Input: part model. Units: mm. Frame: model coordinates. Face numbers are marked on the shaded views. A direction names the side the tool comes from. Round coordinates to 2 decimals unless told otherwise and drop trailing zeros. Loops run counter-clockwise (first coordinate to the right, second up) from the corner with the lowest first, then second, coordinate; pieces in that order, holes last. Notation, with made-up numbers: (35.25, -36.75) -> (91.25, -36.75) arc R27 ccw to (91.25, -10.75) -> close; hole circle Ø10 at (-6, 20). An arc over 180 degrees is marked (long way). Answer in a Markdown table with one row per item. Add a question column.
Q1. Pin query (flat end, axial travel): pin 1 (1.4 mm diameter, centred on x = 8.5, y = 13, fed in from +Z). Return the tip coordinate at first contact, or that it passes through.
Q2. Section C-C, the plane x = 24. Output: boundary loops of the cut face in (y, z).
Q3. Section B-B, the plane y = 14.25. Output: boundary loops of the cut face in (x, z).
Q4. Ray query, L1, parallel to X at y = 5.5, z = 3.25; L2, parallel to Y at x = 7, z = 8.25; L3, parallel to Z at x = 39, y = 7. Return the intervals inside material, ascending. Write a range as from..to.
Q5. Section A-A, the plane z = 5.5. Output: boundary loops of the cut face in (x, y), and give its area (3 significant figures).
Q6. Reachability of the marked faces 1 and 2 from +Z, -Z, +X, -X, +Y, -Y: full face, straight path, thin tool, end or side. Return the list, or none.
Q7. Mould query, pull axis Y, two halves, no side actions, for the marked faces 3, 4, 5 and 6. Classes: pulls with the +Y half, pulls with the -Y half, needs draft (parallel to the pull), parting line crosses it, or undercut.
```python
from build123d import *

# Parameters (mm, degrees)
BOX001_W     = 4.7
BOX001_H     = 11
BOX001_DEPTH = 12
BOX002_W     = 4.7
BOX002_H     = 11
BOX002_DEPTH = 12
BOX_W        = 4.7
BOX_H        = 11
BOX_DEPTH    = 12
BOX003_W     = 45
BOX003_H     = 21
BOX003_DEPTH = 10


with BuildPart() as box001:
    # Box001 → Box001 (new body)
    with BuildSketch(Plane(origin=(15, 0, 0), x_dir=(1, 0, 0), z_dir=(0, 0, 1))):
        with Locations((2.35, 5.5)):
            Rectangle(BOX001_W, BOX001_H)
    extrude(amount=BOX001_DEPTH)


with BuildPart() as box002:
    # Box002 → Box002 (new body)
    with BuildSketch(Plane(origin=(30, 0, 0), x_dir=(1, 0, 0), z_dir=(0, 0, 1))):
        with Locations((2.35, 5.5)):
            Rectangle(BOX002_W, BOX002_H)
    extrude(amount=BOX002_DEPTH)


with BuildPart() as ranuras:
    # Box → Box (new body)
    with BuildSketch(Plane.XY):
        with Locations((2.35, 5.5)):
            Rectangle(BOX_W, BOX_H)
    extrude(amount=BOX_DEPTH)

    # Fusion: union Box001, Box002
    add(box001.part)
    add(box002.part)


with BuildPart() as ranuras_1:
    # Fusion placement: moved
    add(ranuras.part.moved(Location((5, 5, 3))))


with BuildPart() as porta_pendrives:
    # Box003 → Box003 (new body)
    with BuildSketch(Plane.XY):
        with Locations((22.5, 10.5)):
            Rectangle(BOX003_W, BOX003_H)
    extrude(amount=BOX003_DEPTH)

    # Cut: cut Ranuras
    add(ranuras_1.part, mode=Mode.SUBTRACT)


solid = porta_pendrives.part
```
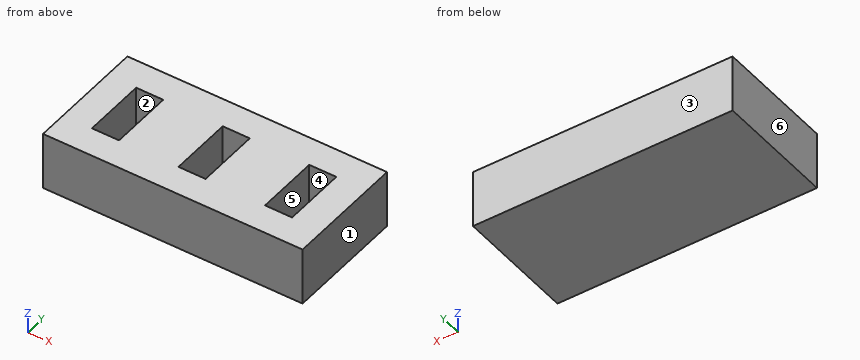
Answer block:
| question | item | result |
|---|---|---|
| 1 | pin 1 | z = 3 |
| 2 | outline | (0, 0) -> (21, 0) -> (21, 10) -> (16, 10) -> (16, 3) -> (5, 3) -> (5, 10) -> (0, 10) -> close |
| 3 | outline | (0, 0) -> (45, 0) -> (45, 10) -> (39.7, 10) -> (39.7, 3) -> (35, 3) -> (35, 10) -> (24.7, 10) -> (24.7, 3) -> (20, 3) -> (20, 10) -> (9.7, 10) -> (9.7, 3) -> (5, 3) -> (5, 10) -> (0, 10) -> close |
| 4 | L1 | 0..5, 9.7..20, 24.7..35, 39.7..45 |
| 4 | L2 | 0..5, 16..21 |
| 4 | L3 | 0..3 |
| 5 | outline | (0, 0) -> (45, 0) -> (45, 21) -> (0, 21) -> close; hole (5, 5) -> (9.7, 5) -> (9.7, 16) -> (5, 16) -> close; hole (20, 5) -> (24.7, 5) -> (24.7, 16) -> (20, 16) -> close; hole (35, 5) -> (39.7, 5) -> (39.7, 16) -> (35, 16) -> close |
| 5 | area | 790 mm^2 |
| 6 | face 1 | +Z, -Z, +X, +Y, -Y |
| 6 | face 2 | +Z |
| 7 | face 3 | pulls with the +Y half |
| 7 | face 4 | undercut |
| 7 | face 5 | undercut |
| 7 | face 6 | needs draft |
